Here's the drawing with two shaded views (mm, measured from the low corner). I have some questions. A direction names the side the tool comes from. Coordinates: 2 decimals unless noted, no trailing zeros. Write each loop counter-clockwise with the first axis right and the second up, starting at its lowest first coordinate (ties: lowest second). Pieces come first, ordered by that corner, then holes.
Item 1: I want a section at D-D on x = 8.5. Please give me the cut outline in (y, z) (3 decimals), then the cut area to 3 significant figures.
Item 2: I want a section at B-B on y = 2.75. Please give me the cut outline in (x, z), then the cut area to 3 significant figures.
Item 3: Thinking about a two-plate mould opening in X: for the marked faces 3, 4 and 5, which applies, +X half, -X half, draft (parallel to the pull), parting line (faces both ways), or undercut?
Item 4: If I drill on probe 1 along X at (y, z) = (3.25, 9.25); probe 2 along X at (y, z) = (4, 14.25); probe 3 along Z at (x, y) = (8.5, 1.5), over which ranges is the centre line in solid material (lowest first)?
Item 5: For P1, Ø2, axis at x = 3, y = 5.5, coming from the +Z side; P2, Ø1.5, axis at x = 18, y = 1.5, coming from the +Z side, each with a flat end and sliding along its axis, tell me the tip position at first contact or that it passes through.
Item 6: I want a section at A-A on z = 12. Please give me the cut outline in (x, y) (3 decimals).
Item 7: I want a section at C-C on x = 15.5. Please give me the cut outline in (y, z) (3 decimals).
Item 8: Which directions (+Z, -Z, +X, -X, +Y, -Y) give clear straight access to the entire face, cutting with the end or side of a thin tool? Please do the marked faces 1 and 2.
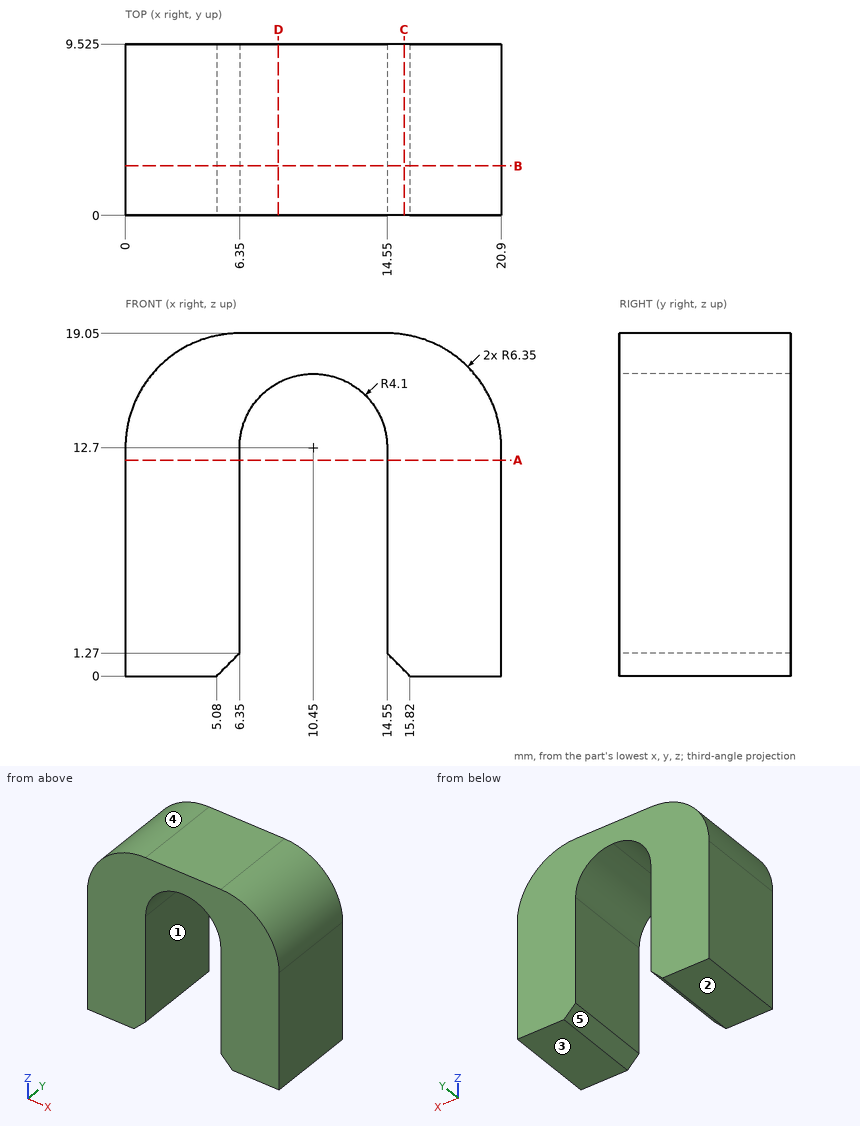
Response values:
1. outline: (0, 16.307) - (9.525, 16.307) - (9.525, 19.05) - (0, 19.05) - close
1. area: 26.1 mm2
2. outline: (0, 0) - (5.08, 0) - (6.35, 1.27) - (6.35, 12.7) arc R4.1 cw to (10.45, 16.8) arc R4.1 cw to (14.55, 12.7) - (14.55, 1.27) - (15.82, 0) - (20.9, 0) - (20.9, 12.7) arc R6.35 ccw to (14.55, 19.05) - (6.35, 19.05) arc R6.35 ccw to (0, 12.7) - close
2. area: 249 mm2
3. face 3: draft
3. face 4: -X half
3. face 5: undercut
4. probe 1: x = 0 to 6.35, 14.55 to 20.9
4. probe 2: x = 0.19 to 6.65, 14.25 to 20.71
4. probe 3: z = 16.31 to 19.05
5. P1: stops at z = 18.6
5. P2: stops at z = 18.45
6. outline: (0, 0) - (6.35, 0) - (6.35, 9.525) - (0, 9.525) - close; (14.55, 0) - (20.9, 0) - (20.9, 9.525) - (14.55, 9.525) - close
7. outline: (0, 0.32) - (9.525, 0.32) - (9.525, 18.979) - (0, 18.979) - close
8. face 1: -Z, +Y, -Y
8. face 2: -Z, +X, -X, +Y, -Y
